Input: part model. Units: mm. Frame: model coordinates. A direction names the side the tool comes from. Coordinates: 2 decimals unless noted, no trailing zeros. Write each loop counter-clockwise with the first axis right and the second up, starting at its lowest first coordinate (ties: lowest second). Pieces come first, ordered by that corner, then holes. Notation, with made-up numbers: M -5.75,56 L 38.25,56 A14 ccw 38.25,72 Z; hole C 33.5,41 d7. An arc over 180 degrees is marked long. Use CSV: the item, a comma, the result in double quotes.
```python
from build123d import *

# Parameters (mm, degrees)
SKETCH_2_W                = 65
SKETCH_2_H                = 35
EXTRUDE_1_DEPTH           = 1
HOLE_WIZARD_3_0_3_1_D     = 3
HOLE_WIZARD_3_0_3_1_DEPTH = 12.4
HOLE_WIZARD_3_0_3_1_TIP   = 0.901290929
SKETCH_5_W                = 18.093294379
SKETCH_5_H                = 8.957076426
EXTRUDE_2_DEPTH           = 4


with BuildPart() as part:
    # 草图2 → 凸台-拉伸1 (new body)
    with BuildSketch(Plane(origin=(0, 0, 0), x_dir=(1, 0, 0), z_dir=(0, 1, 0))):
        Rectangle(SKETCH_2_W, SKETCH_2_H)
    extrude(amount=EXTRUDE_1_DEPTH)

    # Ø3.0 (3) 直径孔1
    with Locations(Plane(origin=(0, 1, 0), x_dir=(1, 0, 0), z_dir=(0, 1, 0))):
        with Locations((-30.5, 15.5), (-30.5, -15.5), (30.5, -15.5), (30.5, 15.5)):
            Hole(HOLE_WIZARD_3_0_3_1_D / 2, depth=HOLE_WIZARD_3_0_3_1_DEPTH)
            with Locations((0, 0, -(HOLE_WIZARD_3_0_3_1_DEPTH + HOLE_WIZARD_3_0_3_1_TIP / 2))):  # 118° drill point
                Cone(0, HOLE_WIZARD_3_0_3_1_D / 2, HOLE_WIZARD_3_0_3_1_TIP, mode=Mode.SUBTRACT)

    # 草图5 → 凸台-拉伸2 (add)
    with BuildSketch(Plane(origin=(0, 1, 0), x_dir=(1, 0, 0), z_dir=(0, 1, 0))):
        with Locations((-0.447853821, -9.89756945)):
            Rectangle(SKETCH_5_W, SKETCH_5_H)
    extrude(amount=EXTRUDE_2_DEPTH)


solid = part.part
```
1. Section D-D (x = -18). Return loops of the section in (y, z).
Resolved:
outline,"M 0,-17.5 L 1,-17.5 L 1,17.5 L 0,17.5 Z"
2. Section B-B (x = 30.5). Return loops of the section in (y, z), then the cut area to 3 significant figures.
Resolved:
outline,"M 0,-17.5 L 1,-17.5 L 1,-17 L 0,-17 Z; M 0,-14 L 1,-14 L 1,14 L 0,14 Z; M 0,17 L 1,17 L 1,17.5 L 0,17.5 Z"
area,"29.0 mm^2"
3. Section A-A (z = 15.5). Return loops of the section in (x, y).
Resolved:
outline,"M -32.5,0 L -32,0 L -32,1 L -32.5,1 Z; M -29,0 L 29,0 L 29,1 L -29,1 Z; M 32,0 L 32.5,0 L 32.5,1 L 32,1 Z"
4. Access query for faces 4 (the flat face through (-1, 3, 14.376)), 5 (the flat face through (-9.495, 3, 10)), 6 (the flat face through (8.599, 3, 10)). Directions: +Z, -Z, +X, -X, +Y, -Y. A direction counts if a zero-diameter tool reaches every point of the face in a straight line with its end or side. Return the directions, or none.
Resolved:
face 4,"+Z, +X, -X, +Y"
face 5,"+Z, -Z, -X, +Y"
face 6,"+Z, -Z, +X, +Y"
5. Section C-C (z = 10.5). Return loops of the section in (x, y).
Resolved:
outline,"M -32.5,0 L 32.5,0 L 32.5,1 L 8.6,1 L 8.6,5 L -9.49,5 L -9.49,1 L -32.5,1 Z"
6. Contact query for flat-ended pins moving along their axis: pin 1 Ø1.2 at (y, z) = (2.5, 8) entering from +X; pin 2 Ø3 at (y, z) = (3, 10.5) entering from -X; pin 3 Ø1.5 at (x, y) = (5, 2) entering from -Z. Output: stop coordinate, or through.
Resolved:
pin 1,"stops at x = 8.6"
pin 2,"stops at x = -9.49"
pin 3,"stops at z = 5.42"
7. Mould query, pull axis Z, two halves, no side actions, for faces 1 (the flat face through (-1, 3, 5.419)), 2 (the cylindrical face through (-29, 0.49, 15.43)), 3 (the flat face through (0, 0, 0)). Classes: pulls with the +Z half, pulls with the -Z half, needs draft (parallel to the pull), parting line crosses it, or undercut.
Resolved:
face 1,"pulls with the -Z half"
face 2,"undercut"
face 3,"needs draft"
8. Material intervals for line 1 (X direction, y = 0.3, z = 15.5); line 2 (Z direction, x = -30.5, y = 0.65); line 3 (Y direction, x = -24, z = -10.5), sorted ascending. Write a range as [from, to].
Resolved:
line 1,"x = [-32.5, -32], [-29, 29], [32, 32.5]"
line 2,"z = [-17.5, -17], [-14, 14], [17, 17.5]"
line 3,"y = [0, 1]"
